from build123d import *

# Parameters (mm, degrees)
RESSALTO_EXTRUS_O1_DEPTH = 15
ESBO_O3_R                = 2.5
CORTE_EXTRUS_O1_DEPTH    = 15
CHANFRO1_SIZE            = 2
FILETE1_R                = 0.5
FILETE2_R                = 0.94
RESSALTO_EXTRUS_O3_DEPTH = 15
CHANFRO5_SIZE            = 2
CHANFRO4_SIZE            = 1


with BuildPart() as part:
    # Esboço1 → Ressalto-extrusão1 (new body)
    with BuildSketch(Plane.XY):
        with BuildLine():
            Line((11, 14.25), (-5, 14.25))
            Line((-5, 14.25), (-5, 4.25))
            Line((-5, 4.25), (1, 4.25))
            Line((1, 4.25), (1, -0.75))
            Line((1, -0.75), (-5, -0.75))
            Line((-5, -0.75), (-5, -17.25))
            Line((-5, -17.25), (15, -17.25))
            Line((15, -17.25), (15, -22.25))
            Line((15, -22.25), (-10, -22.25))
            Line((-10, -22.25), (-10, 19.25))
            Line((-10, 19.25), (6, 19.25))
            Line((6, 19.25), (6, 16.25))
            Line((6, 16.25), (10.504380809, 16.25))
            ThreePointArc((10.504380809, 16.25), (10.676386068, 16.357306387), (10.826229508, 16.493861918))
            ThreePointArc((10.826229508, 16.493861918), (10.936214298, 16.519561844), (11, 16.426349589))
            Line((11, 16.426349589), (11, 16.25))
            Line((11, 16.25), (11, 14.25))
        make_face()
    extrude(amount=RESSALTO_EXTRUS_O1_DEPTH)

    # Esboço3 → Corte-extrusão1 (cut)
    with BuildSketch(Plane.XZ.offset(22.25)):
        with Locations(Location((7, 7.5, 0), (0, 0, 270))):
            Circle(ESBO_O3_R)
    extrude(amount=-CORTE_EXTRUS_O1_DEPTH, mode=Mode.SUBTRACT)

    # Chanfro1
    chanfro1_edges = [part.edges().sort_by_distance(p)[0] for p in [
        (7, -22.25, 10),
    ]]
    chamfer(chanfro1_edges, length=CHANFRO1_SIZE)

    # Filete1
    filete1_edges = [part.edges().sort_by_distance(p)[0] for p in [
        (7, -17.25, 10),
    ]]
    fillet(filete1_edges, radius=FILETE1_R)

    # Filete2
    filete2_edges = [part.edges().sort_by_distance(p)[0] for p in [
        (6, 16.25, 7.5),
    ]]
    fillet(filete2_edges, radius=FILETE2_R)

    # Esboço5 → Ressalto-extrusão3 (add)
    with BuildSketch(Plane.XY.offset(15)):
        Polygon((6, 19.25), (6, 21.25), (4, 21.25), (2, 19.25), align=None)
    extrude(amount=-RESSALTO_EXTRUS_O3_DEPTH)

    # Chanfro5
    chanfro5_edges = [part.edges().sort_by_distance(p)[0] for p in [
        (15, -22.25, 7.5),
        (-10, -22.25, 7.5),
        (-10, 19.25, 7.5),
        (1, 4.25, 7.5),
    ]]
    chamfer(chanfro5_edges, length=CHANFRO5_SIZE)

    # Chanfro4
    chanfro4_edges = [part.edges().sort_by_distance(p)[0] for p in [
        (-5, 9.25, 15),
        (-2, -0.75, 0),
        (3, 14.25, 15),
        (-5, -9, 0),
        (5, -17.25, 0),
        (3, 14.25, 0),
        (-5, 9.25, 0),
        (11, 14.25, 7.5),
        (5, -17.25, 15),
        (-5, -9, 15),
        (-2, -0.75, 15),
        (-3, 19.25, 0),
        (-3, 19.25, 15),
        (5, 21.25, 15),
        (3, 20.25, 15),
        (3, 20.25, 0),
        (5, 21.25, 0),
        (-3, 4.25, 0),
        (-3, 4.25, 15),
        (15, -18.75, 0),
        (2.5, -22.25, 0),
        (-10, -1.5, 0),
        (-9, 18.25, 0),
        (-9, -21.25, 0),
        (14, -21.25, 0),
        (-10, -1.5, 15),
        (2.5, -22.25, 15),
        (15, -18.75, 15),
        (-9, 18.25, 15),
        (-9, -21.25, 15),
        (14, -21.25, 15),
    ]]
    chamfer(chanfro4_edges, length=CHANFRO4_SIZE)


solid = part.part
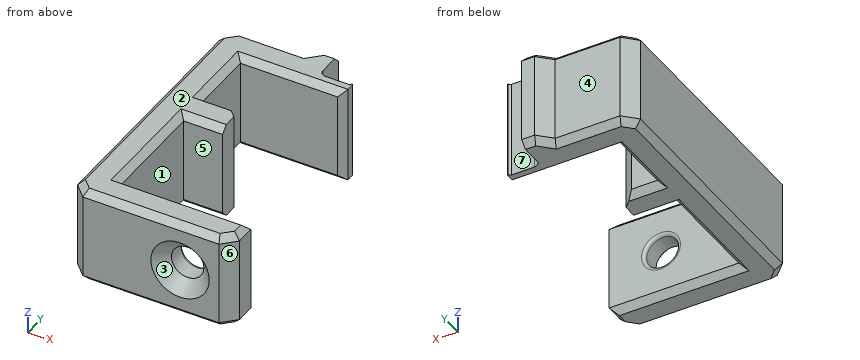
Can you work these out from the model? Positions are in its coordinate system, mm. Face numbers are marked on the shaded views. A direction names the side the tool comes from. Round coordinates to 2 decimals unless told otherwise and drop trailing zeros. Write each loop counter-clockwise with the first axis right and the second up, starting at its lowest first coordinate (ties: lowest second). Pieces come first, ordered by that corner, then holes. Notation, with made-up numbers: M 34,-32 L 70,-32 A21 ccw 70,-6 Z; hole C 78.5,-24.5 d9. An arc over 180 degrees is marked long. Use a Markdown table: item, result.
Item 1: We'd pull the mould along Z, two halves only. Please class the marked faces 1, 2 and 3: released by +Z, released by -Z, zero draft, split by the parting line, or undercut.
Found:
| item | result |
|---|---|
| face 1 | zero draft |
| face 2 | released by +Z |
| face 3 | undercut |
Item 2: I want a section at A-A (x = -2.25). List the corners of the cut face in (y, z) for me, and give its area (3 significant figures).
Found:
| item | result |
|---|---|
| outline | M -22.25,1 L -21.25,0 L -18.25,0 L -17.25,1 L -17.25,14 L -18.25,15 L -21.25,15 L -22.25,14 Z; M -0.75,1 L 0.25,0 L 3.25,0 L 4.25,1 L 4.25,14 L 3.25,15 L 0.25,15 L -0.75,14 Z; M 14.25,1 L 15.25,0 L 18.25,0 L 19.25,1 L 19.25,14 L 18.25,15 L 15.25,15 L 14.25,14 Z |
| area | 219 mm2 |
Item 3: If I drill on line 1 along Y through (x, z) = (7, 1.75); line 2 along X through (y, z) = (-19.05, 7.5); line 3 along Y through (x, z) = (5.75, 13.5), over which ranges is the centre line in solid material (lowest first)? Write a range as [from, to].
Found:
| item | result |
|---|---|
| line 1 | y = [-22.25, -17.25], [14.25, 16.25] |
| line 2 | x = [-10, 4.5], [9.5, 15] |
| line 3 | y = [-22.25, -17.25], [14.25, 21.25] |
Item 4: I want a section at C-C (z = 13). List the corners of the cut face in (x, y) for me.
Found:
| item | result |
|---|---|
| outline | M -10,-20.25 L -8,-22.25 L 13,-22.25 L 15,-20.25 L 15,-17.25 L -5,-17.25 L -5,-0.75 L 1,-0.75 L 1,2.25 L -1,4.25 L -5,4.25 L -5,14.25 L 10,14.25 L 11,15.25 L 11,16.43 A0.1 ccw 10.83,16.49 A1.12 cw 10.5,16.25 L 6.94,16.25 A0.94 cw 6,17.19 L 6,21.25 L 4,21.25 L 2,19.25 L -8,19.25 L -10,17.25 Z |
Item 5: For pin 1 Ø6.5 at (y, z) = (-10.5, 6.5) entering from +X; pin 2 Ø6 at (x, z) = (7, 7.5) entering from +Y; pin 3 Ø1.5 at (x, z) = (8.5, 13) entering from +Y; pin 4 Ø3 at (x, z) = (9.5, 7.5) entering from +Y, each with a flat end and sliding along its axis, tell me the tip position at first contact or that it passes through.
Found:
| item | result |
|---|---|
| pin 1 | stops at x = -5 |
| pin 2 | stops at y = 21.25 |
| pin 3 | stops at y = 16.25 |
| pin 4 | stops at y = 16.53 |
Item 6: Which directions (+Z, -Z, +X, -X, +Y, -Y) give clear straight access to the entire face, cutting with the end or side of a thin tool? Please do the marked faces 4, 5, 6 and 7.
Found:
| item | result |
|---|---|
| face 4 | +Z, -Z, -X, +Y |
| face 5 | +Z, -Z, +X |
| face 6 | +Z, -Z, +X, -Y |
| face 7 | +Z, -Z, +Y |
Item 7: I want a section at D-D (y = 6.5). List the corners of the cut face in (x, z) for me, and give its area (3 significant figures).
Found:
| item | result |
|---|---|
| outline | M -10,1 L -9,0 L -6,0 L -5,1 L -5,14 L -6,15 L -9,15 L -10,14 Z |
| area | 73.0 mm2 |
